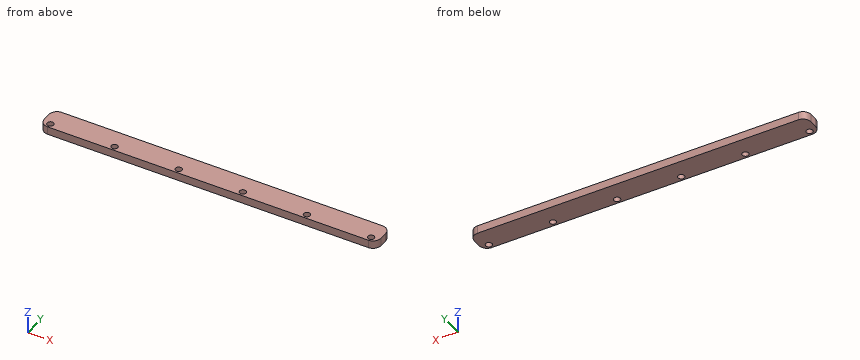
```python
from build123d import *

# Parameters (mm, degrees)
ESQUISSE1_W        = 210
ESQUISSE1_H        = 15
ESQUISSE1_R        = 2
BOSS_EXTRU_1_DEPTH = 5
CONG_1_R           = 5


with BuildPart() as part:
    # Esquisse1 → Boss.-Extru.1 (new body)
    with BuildSketch(Plane.XY):
        with Locations((105, 7.5)):
            Rectangle(ESQUISSE1_W, ESQUISSE1_H)
        with Locations((5, 3)):
            Circle(ESQUISSE1_R, mode=Mode.SUBTRACT)
        with Locations((45, 3)):
            Circle(ESQUISSE1_R, mode=Mode.SUBTRACT)
        with Locations((85, 3)):
            Circle(ESQUISSE1_R, mode=Mode.SUBTRACT)
        with Locations((125, 3)):
            Circle(ESQUISSE1_R, mode=Mode.SUBTRACT)
        with Locations((165, 3)):
            Circle(ESQUISSE1_R, mode=Mode.SUBTRACT)
        with Locations((205, 3)):
            Circle(ESQUISSE1_R, mode=Mode.SUBTRACT)
    extrude(amount=BOSS_EXTRU_1_DEPTH)

    # Congé1
    cong_1_edges = [part.edges().sort_by_distance(p)[0] for p in [
        (0, 15, 2.5),
        (210, 15, 2.5),
        (210, 0, 2.5),
        (0, 0, 2.5),
    ]]
    fillet(cong_1_edges, radius=CONG_1_R)


solid = part.part
```
Work out the finished part from the listing and answer in its coordinate system (mm). Round coordinates to 2 decimals unless told otherwise and drop trailing zeros. Loops run counter-clockwise (first coordinate to the right, second up) from the corner with the lowest first, then second, coordinate; pieces in that order, holes last.
(1) The part is cut by section B-B, the plane z = 3.45. Give the vertices of the cut face in (x, y).
Computed values:
outline: (0, 5) arc R5 ccw to (5, 0) - (205, 0) arc R5 ccw to (210, 5) - (210, 10) arc R5 ccw to (205, 15) - (5, 15) arc R5 ccw to (0, 10) - close; hole circle Ø4 at (5, 3); hole circle Ø4 at (45, 3); hole circle Ø4 at (85, 3); hole circle Ø4 at (125, 3); hole circle Ø4 at (165, 3); hole circle Ø4 at (205, 3)
(2) This flat-tipped pin is pushed along its axis until it touches: P1, Ø3, axis at y = 13, z = 1.5, coming from the -X side. Where does it stop, or does it pass through?
Computed values:
P1: stops at x = 0.23
(3) Find the intervals of material crossed by L1, parallel to Y at x = 45, z = 4; L2, parallel to Y at x = 84, z = 3.7; L3, parallel to X at y = 12.5, z = 4.45, in increasing order.
Computed values:
L1: y = 0 to 1, 5 to 15
L2: y = 0 to 1.27, 4.73 to 15
L3: x = 0.67 to 209.33
(4) The part is cut by section A-A, the plane x = 125. Give the vertices of the cut face in (y, z), and give its area (3 significant figures).
Computed values:
outline: (0, 0) - (1, 0) - (1, 5) - (0, 5) - close; (5, 0) - (15, 0) - (15, 5) - (5, 5) - close
area: 55.0 mm2
